Input: part model. Units: mm. Frame: model coordinates. A direction names the side the tool comes from. Round coordinates to 2 decimals unless told otherwise and drop trailing zeros. Loops run counter-clockwise (first coordinate to the right, second up) from the corner with the lowest first, then second, coordinate; pieces in that order, holes last.
(1) Line query: line 1 (X direction, y = 20.75, z = 9.5); line 2 (X direction, y = 16.5, z = 14.25); line 3 (Z direction, x = -4.5, y = 24). Output: solid intervals per line, ascending.
(2) Access query for faces 4 (the face through (-15.34, 9.86, 0.855)), 5 (the face through (-15.34, 9.86, 19.145)), 6 (the face through (-34.438, 10, 10)), 7 (the face through (-33.58, 10.14, 19.1)), 8 (the face through (-33.58, 10.14, 0.9)). Directions: +Z, -Z, +X, -X, +Y, -Y. A direction counts if a zero-diameter tool reaches every point of the face in a straight line with its end or side. Return the directions, or none.
(3) Draft query along Y for faces 1 (the face through (-24, 25, 10)), 2 (the face through (-14.438, 10, 10)), 3 (the face through (-25.089, 14.957, 10.14)). Return one class per face: released by +Y, released by -Y, zero draft, split by the parting line, or undercut.
(4) Cut plane C-C, the plane y = 10. Output: boundary loops of the cut face in (x, z).
(5) Cut plane D-D, the plane x = -25. Output: boundary loops of the cut face in (y, z), and give its area (3 significant figures).
(6) Cut plane B-B, the plane z = 5.25. Output: boundary loops of the cut face in (x, y).
(7) First-contact query: pin 1 Ø1.5 at (y, z) = (5.5, 5) entering from +X; pin 2 Ø3 at (x, z) = (-41.5, 6.5) entering from -Y; pin 3 Ø12 at (x, y) = (-9.5, 12) entering from -Z. Flat tips, straight axial feed; report the tip coordinate or a pass-through.
(8) Cut plane A-A, the plane z = 10. Output: boundary loops of the cut face in (x, y), and give its area (3 significant figures).
from build123d import *

# Parameters (mm, degrees)
AUFSATZ_LINEAR_AUSTRAGEN1_DEPTH = 20
SKIZZE2_R                       = 5
SCHNITT_LINEAR_AUSTRAGEN1_DEPTH = 20
SKIZZE3_R                       = 2.75
SCHNITT_LINEAR_AUSTRAGEN2_DEPTH = 20
VERRUNDUNG1_R                   = 3


with BuildPart() as part:
    # Skizze1 → Aufsatz-Linear austragen1 (new body)
    with BuildSketch(Plane.XY):
        Polygon((-34.43835366, 0), (-34.43835366, 20), (-49.43835366, 20), (-49.43835366, 25), (-24.43835366, 25), (0.56164634, 25), (0.56164634, 20), (-14.43835366, 20), (-14.43835366, 0), (-24.43835366, 0), align=None)
    extrude(amount=AUFSATZ_LINEAR_AUSTRAGEN1_DEPTH)

    # Skizze2 → Schnitt-Linear austragen1 (cut)
    with BuildSketch(Plane.XY.offset(20)):
        with Locations((-24.43835366, 10)):
            Circle(SKIZZE2_R)
    extrude(amount=-SCHNITT_LINEAR_AUSTRAGEN1_DEPTH, mode=Mode.SUBTRACT)

    # Skizze3 → Schnitt-Linear austragen2 (cut)
    with BuildSketch(Plane(origin=(0, 25, 0), x_dir=(1, 0, 0), z_dir=(0, 1, 0))):
        with Locations(Location((-41.93835366, -10, 0), (0, 0, 180))):
            Circle(SKIZZE3_R)
        with Locations(Location((-6.93835366, -10, 0), (0, 0, 180))):
            Circle(SKIZZE3_R)
    extrude(amount=-SCHNITT_LINEAR_AUSTRAGEN2_DEPTH, mode=Mode.SUBTRACT)

    # Verrundung1
    verrundung1_edges = [part.edges().sort_by_distance(p)[0] for p in [
        (-14.43835366, 10, 20),
        (-14.43835366, 10, 0),
        (-34.43835366, 10, 20),
        (-34.43835366, 10, 0),
    ]]
    fillet(verrundung1_edges, radius=VERRUNDUNG1_R)


solid = part.part
Reported:
1. line 1: x = -49.44 to -44.64, -39.23 to -9.64, -4.23 to 0.56
1. line 2: x = -34.44 to -14.44
1. line 3: z = 0 to 8.73, 11.27 to 20
2. face 4: -Z, +X, -Y
2. face 5: +Z, +X, -Y
2. face 6: +Z, -Z, -X, -Y
2. face 7: +Z, -X, -Y
2. face 8: -Z, -X, -Y
3. face 1: released by +Y
3. face 2: zero draft
3. face 3: undercut
4. outline: (-34.44, 3) arc R3 ccw to (-31.44, 0) - (-29.44, 0) - (-29.44, 20) - (-31.44, 20) arc R3 ccw to (-34.44, 17) - close; (-19.44, 0) - (-17.44, 0) arc R3 ccw to (-14.44, 3) - (-14.44, 17) arc R3 ccw to (-17.44, 20) - (-19.44, 20) - close
5. outline: (0, 0) - (5.03, 0) - (5.03, 20) - (0, 20) - close; (14.97, 0) - (25, 0) - (25, 20) - (14.97, 20) - close
5. area: 301 mm2
6. outline: (-49.44, 20) - (-34.44, 20) - (-34.44, 0) - (-14.44, 0) - (-14.44, 20) - (0.56, 20) - (0.56, 25) - (-49.44, 25) - close; hole circle Ø10 at (-24.44, 10)
7. pin 1: stops at x = -14.44
7. pin 2: stops at y = 20
7. pin 3: stops at z = 0.71
8. outline: (-49.44, 20) - (-44.69, 20) - (-44.69, 25) - (-49.44, 25) - close; (-39.19, 20) - (-34.44, 20) - (-34.44, 0) - (-14.44, 0) - (-14.44, 20) - (-9.69, 20) - (-9.69, 25) - (-39.19, 25) - close; (-4.19, 20) - (0.56, 20) - (0.56, 25) - (-4.19, 25) - close; hole circle Ø10 at (-24.44, 10)
8. area: 516 mm2
